from build123d import *

# Parameters (mm, degrees)
EXTRUDE_1_DEPTH = 4


with BuildPart() as part:
    # 草图1 → 凸台-拉伸1 (new body)
    with BuildSketch(Plane(origin=(0, 0, 0), x_dir=(1, 0, 0), z_dir=(0, 1, 0))):
        with BuildLine():
            Line((-19.428200902, -5.776577465), (-24.227594621, -5.776577465))
            Line((-24.227594621, -5.776577465), (-24.227594621, -1.535252783))
            Line((-24.227594621, -1.535252783), (-28.134077881, -1.535252783))
            Line((-28.134077881, -1.535252783), (-28.134077881, 0.585409558))
            Line((-28.134077881, 0.585409558), (-33.603154445, 0.585409558))
            Line((-33.603154445, 0.585409558), (-41.750962387, -47.296913826))
            Line((-41.750962387, -47.296913826), (-43.536783306, -47.296913826))
            Line((-43.536783306, -47.296913826), (-46.636151448, -65.511008799))
            Line((-46.636151448, -65.511008799), (8.433030865, -65.511008799))
            Line((8.433030865, -65.511008799), (8.433030865, -51.611008799))
            Line((8.433030865, -51.611008799), (16.433030865, -51.611008799))
            Line((16.433030865, -51.611008799), (16.433030865, -65.511008799))
            Line((16.433030865, -65.511008799), (68.300251733, -65.511008799))
            Line((68.300251733, -65.511008799), (65.286678932, -47.296913826))
            Line((65.286678932, -47.296913826), (63.500858013, -47.296913826))
            Line((63.500858013, -47.296913826), (55.578594097, 0.585409558))
            Line((55.578594097, 0.585409558), (49.7723597, 0.585409558))
            Line((49.7723597, 0.585409558), (49.7723597, -1.535252783))
            Line((49.7723597, -1.535252783), (46.089104055, -1.535252783))
            Line((46.089104055, -1.535252783), (46.089104055, -5.776577465))
            Line((46.089104055, -5.776577465), (41.512937951, -5.776577465))
            add(Edge.make_bspline(
                [(41.512937951, -5.776577465), (42.69533512, -10.410562899), (50.01726791, -6.582058067), (51.893022041, -11.245654029)],
                knots=[0, 0, 0, 0, 1, 1, 1, 1], degree=3))
            Line((51.893022041, -11.245654029), (57.808553835, -47.296913826))
            Line((57.808553835, -47.296913826), (-35.835430593, -47.296913826))
            Line((-35.835430593, -47.296913826), (-30.031512607, -11.245654029))
            add(Edge.make_bspline(
                [(-19.428200902, -5.776577465), (-21.07412713, -10.350937498), (-27.778264505, -6.819763811), (-30.031512607, -11.245654029)],
                knots=[0, 0, 0, 0, 1, 1, 1, 1], degree=3))
        make_face()
    extrude(amount=EXTRUDE_1_DEPTH)


solid = part.part
Geometry check sheet. Reference: the model listing, model coordinates, mm. A direction names the side the tool comes from. Round coordinates to 2 decimals unless told otherwise and drop trailing zeros. Order: outer loops, then holes, each group sorted by start corner. A loop starts at its lowest first (then second) coordinate and runs counter-clockwise, first axis right, second up. Notation, with made-up numbers: M -5,37.25 L -1,37.25 A20 ccw -1,58.25 Z; hole C 3,78 d5. An arc over 180 degrees is marked long. Write each question's results on one line, items separated by ' | '. Start each with the question number.
1. Go/stop test with flat-tipped pins: P1, Ø0.6, axis at y = 2, z = 1, coming from the -X side; P2, Ø2, axis at y = 2.5, z = 60.5, coming from the +X side; P3, Ø1.1, axis at x = 47.5, y = 2.5, coming from the -Z side. Record where each tip stops, or that it passes through.
2. Set-up check for faces 5 (the face through (48, 2, 1.535)), 6 (the face through (12, 2, 47.297)), 7 (the face through (-45.065, 1.972, 56.276)), 8 (the face through (16.433, 2, 58)): record each of +Z, -Z, +X, -X, +Y, -Y from which the full face is reachable in a straight line by a thin tool's end or side.
3. Draft check along Z on faces 1 (the face through (-19, 2, 65.511)), 2 (the face through (54.81, 1.97, 29.02)), 3 (the face through (59.595, 1.972, 23.691)), 4 (the face through (15, 4, 49)). Enter one of: pulls with the +Z half, pulls with the -Z half, needs draft (parallel to the pull), parting line crosses it, or undercut.
4. Cross-section at C-C on x = -17.5. Record the boundary of the cut face in (y, z), plus the area to 3 significant figures.
5. Cross-section at A-A on z = 13. Record the boundary of the cut face in (x, y), plus the area to 3 significant figures.
6. Cross-section at B-B on z = 4.5. Record the boundary of the cut face in (x, y), plus the area to 3 significant figures.
7. Material ranges on L1, parallel to Z at x = -10, y = 0.2; L2, parallel to X at y = 1.8, z = 54.5; L3, parallel to X at y = 0.25, z = 34.5, recorded low to high. Write a range as from..to.
Resolved:
1) P1: x = -33.92 | P2: x = 67.64 | P3: z = 1.54
2) face 5: -Z, +Y, -Y | face 6: +Y, -Y | face 7: -Z, -X, +Y, -Y | face 8: +Z, +Y, -Y
3) face 1: pulls with the +Z half | face 2: undercut | face 3: pulls with the -Z half | face 4: needs draft
4) outline: M 0,47.3 L 4,47.3 L 4,65.51 L 0,65.51 Z | area: 72.9 mm2
5) outline: M -35.91,0 L -30.31,0 L -30.31,4 L -35.91,4 Z; M 52.18,0 L 57.83,0 L 57.83,4 L 52.18,4 Z | area: 45.0 mm2
6) outline: M -34.47,0 L -24.23,0 L -24.23,4 L -34.47,4 Z; M 46.09,0 L 56.42,0 L 56.42,4 L 46.09,4 Z | area: 82.3 mm2
7) L1: 47.3..65.51 | L2: -44.76..8.43, 16.43..66.48 | L3: -39.57..-33.78, 55.71..61.38
